Design review of the part shown in the three views and the two pictorial views. Dimensions are in mm from the part's minimum x, y and z. Give positions to 0.01 mm unless a question says otherwise; leave off trailing zeros. Loops run counter-clockwise (first coordinate to the right, second up) from the corner with the lowest first, then second, coordinate; pieces in that order, holes last. Notation, with made-up numbers: (-2.75, 78) - (1.25, 78) arc R33 ccw to (1.25, 109) - close; hole circle Ø5 at (25, 59). An arc over 180 degrees is marked (long way). Answer in a Markdown table with one row per item.
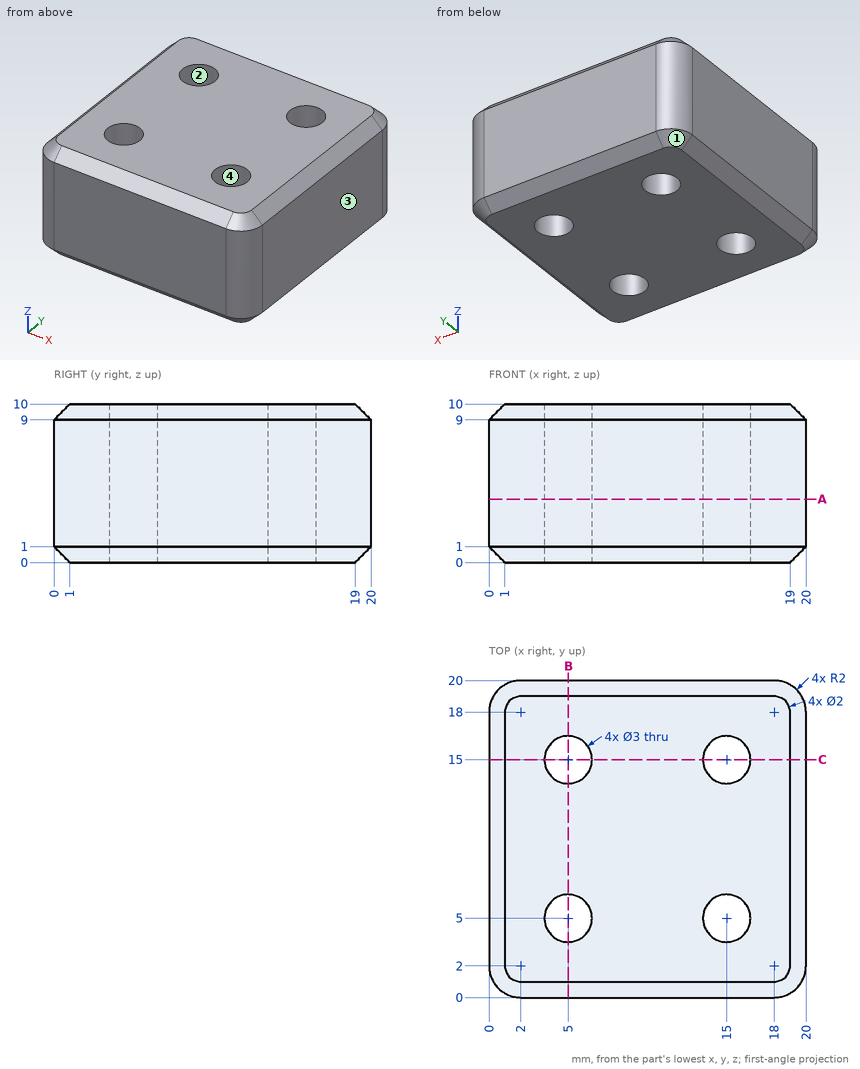
1. Clearance check with a flat-ended pin moving along its axis: pin 1 (2.5 mm diameter, centred on x = 15, y = 5, fed in from -Z). State where the tip first meets the part, or that it passes through.
Values:
| item | result |
|---|---|
| pin 1 | passes through |
2. We need section A-A, the plane z = 4. Give the boundary of the cut face in (x, y), and give its area (3 significant figures).
Values:
| item | result |
|---|---|
| outline | (0, 2) arc R2 ccw to (2, 0) - (18, 0) arc R2 ccw to (20, 2) - (20, 18) arc R2 ccw to (18, 20) - (2, 20) arc R2 ccw to (0, 18) - close; hole circle Ø3 at (5, 5); hole circle Ø3 at (5, 15); hole circle Ø3 at (15, 5); hole circle Ø3 at (15, 15) |
| area | 368 mm^2 |
3. Wall thickness on line 1 (Y direction, x = 15, z = 7.75); line 2 (X direction, y = 14.5, z = 3.25); line 3 (X direction, y = 4.75, z = 8.25): over which ranges is each line inside the solid? List them lowest first. Write a range as [from, to].
Values:
| item | result |
|---|---|
| line 1 | y = [0, 3.5], [6.5, 13.5], [16.5, 20] |
| line 2 | x = [0, 3.59], [6.41, 13.59], [16.41, 20] |
| line 3 | x = [0, 3.52], [6.48, 13.52], [16.48, 20] |
4. We need section B-B, the plane x = 5. Give the boundary of the cut face in (y, z), and give its area (3 significant figures).
Values:
| item | result |
|---|---|
| outline | (0, 1) - (1, 0) - (3.5, 0) - (3.5, 10) - (1, 10) - (0, 9) - close; (6.5, 0) - (13.5, 0) - (13.5, 10) - (6.5, 10) - close; (16.5, 0) - (19, 0) - (20, 1) - (20, 9) - (19, 10) - (16.5, 10) - close |
| area | 138 mm^2 |
5. Mouldability with a two-part tool opening along X and no side actions: class the marked faces 1, 2, 3 and 4 as released by +X, released by -X, zero draft, split by the parting line, or undercut.
Values:
| item | result |
|---|---|
| face 1 | released by -X |
| face 2 | undercut |
| face 3 | released by +X |
| face 4 | undercut |
